```python
from build123d import *

# Parameters (mm, degrees)
F3_D = 13.49248


with BuildPart() as f1:
    # F0 (on Front) → F1 (revolve)
    with BuildSketch(Plane.XZ):
        Polygon((41.275, 0), (44.45, 0), (44.45, 1.5875), (85.725, 1.5875), (85.725, 9.525), (85.725, 14.2875), (81.0895, 14.2875), (81.0895, 9.525), (57.15, 9.525), (57.15, 4.7625), (41.275, 4.7625), align=None)
    revolve(axis=Axis((0, 0, 11.4762624726), (0, 0, -1)))

    # F3 (through all)
    with Locations(Plane(origin=(0, 0, 1.5875), x_dir=(1, 0, 0), z_dir=(0, 0, -1))):
        with Locations((0, 65.0875), (-46.0238126205, 46.0238126205), (-65.0875, 0), (-46.0238126205, -46.0238126205), (0, -65.0875), (46.0238126205, -46.0238126205), (65.0875, 0), (46.0238126205, 46.0238126205)):
            Hole(F3_D / 2)


solid = f1.part
```
The model under review builds one solid part; all positions refer to its coordinate system, in mm. A direction names the side the tool comes from. Round coordinates to 2 decimals unless told otherwise and drop trailing zeros. Loops run counter-clockwise (first coordinate to the right, second up) from the corner with the lowest first, then second, coordinate; pieces in that order, holes last. Notation, with made-up numbers: (-37.5, 84.5) - (16.5, 84.5) arc R22 cw to (16.5, 112.5) - close; hole circle Ø1 at (-11, 21.5). An arc over 180 degrees is marked (long way). Write each question's results on one line, items separated by ' | '. Start each with the question number.
Q1. Take a section at A-A on x = 0. Give the number of separate pieces and of enclosed holes in the cut face, plus the area to 3 significant figures.
Q2. Take a section at D-D on x = -49.5. Give the boundary of the cut face in (y, z) (1 decimal), plus the area to 3 significant figures.
Q3. Insertion check: P1, Ø21.5, axis at x = 0, y = 65.09, coming from the +Z side (3 decimals); P2, Ø11, axis at x = 0, y = -65.09, coming from the -Z side; P3, Ø1, axis at y = -39, z = 4.5, coming from the -X side; P4, Ø1, axis at y = 61.5, z = 1.5, coming from the +X side. Each pin has a flat end and moves straight along its axis. Give the tip position at first contact, or say it passes through.
Q4. Draft analysis for pull direction X (two halves, no side actions). For faces 1 (the cylindrical face through (42.397, -13.352, 0.805)), 2 (the flat face through (-29.4, 29.4, 0)), 3 (the cylindrical face through (1.462, 71.673, 5.612)), state which applies: pulls with the +X half, pulls with the -X half, needs draft (parallel to the pull), parting line crosses it, or undercut.
Q5. Wall thickness on line 1 along Y through (x, z) = (0, 6.75) (3 decimals); line 2 along Y through (x, z) = (41, 9.25); line 3 along Z through (x, y) = (45, -25.5): over which ranges is each line inside the solid? List them lowest first. Write a range as [from, to].
Q6. Take a section at C-C on y = -21.5. Give the boundary of the cut face in (x, z) (1 decimal).
Q7. Tool access review of faces 4 (the cylindrical face through (-49.651, 40.335, 5.612)), 5 (the flat face through (-37, 37, 1.588)), 6 (the flat face through (-55, -19, 9.525)): name each direction out of +Z, -Z, +X, -X, +Y, -Y from which nothing blocks a thin tool from reaching the whole face with its end or side.
Data:
1) separate pieces: 4 | enclosed holes: 0 | area: 394 mm²
2) outline: (-70, 1.6) - (-51.8, 1.6) - (-51.8, 9.5) - (-64.2, 9.5) - (-64.2, 14.3) - (-70, 14.3) - close; (-40.2, 1.6) - (40.2, 1.6) - (40.2, 9.5) - (28.6, 9.5) - (28.6, 4.8) - (-28.6, 4.8) - (-28.6, 9.5) - (-40.2, 9.5) - close; (51.8, 1.6) - (70, 1.6) - (70, 14.3) - (64.2, 14.3) - (64.2, 9.5) - (51.8, 9.5) - close | area: 710 mm²
3) P1: stops at z = 9.525 | P2: passes through | P3: stops at x = -76.59 | P4: stops at x = 60.22
4) face 1: parting line crosses it | face 2: needs draft | face 3: undercut
5) line 1: y = [-85.725, -71.834], [-58.341, -57.15], [57.15, 58.341], [71.834, 85.725] | line 2: y = [-75.28, -50.53], [-41.52, -39.81], [39.81, 41.52], [50.53, 75.28] | line 3: z = [1.59, 4.76]
6) outline: (-83, 1.6) - (-38.9, 1.6) - (-38.9, 0) - (-35.2, 0) - (-35.2, 4.8) - (-53, 4.8) - (-53, 9.5) - (-78.2, 9.5) - (-78.2, 14.3) - (-83, 14.3) - close; (35.2, 0) - (38.9, 0) - (38.9, 1.6) - (83, 1.6) - (83, 14.3) - (78.2, 14.3) - (78.2, 9.5) - (53, 9.5) - (53, 4.8) - (35.2, 4.8) - close
7) face 4: +Z, -Z | face 5: -Z | face 6: +Z
